```python
from build123d import *

# Parameters (mm, degrees)
SKETCH1_R            = 7.5
BOSS_EXTRUDE1_DEPTH  = 25
SKETCH4_R            = 7.5
BOSS_EXTRUDE4_DEPTH  = 40
BOSS_EXTRUDE4_TAPER  = 5
SKETCH5_R            = 2
BOSS_EXTRUDE5_DEPTH  = 1
SKETCH5_5_R          = 1.5
BOSS_EXTRUDE6_DEPTH  = 5
SKETCH6_R            = 2
BOSS_EXTRUDE7_DEPTH  = 1
SKETCH8_R            = 1.5
BOSS_EXTRUDE8_DEPTH  = 1
SKETCH9_R            = 2
BOSS_EXTRUDE9_DEPTH  = 1
SKETCH10_W           = 0.5
SKETCH10_H           = 3
BOSS_EXTRUDE10_DEPTH = 2
SKETCH11_W           = 0.5
SKETCH11_H           = 2
BOSS_EXTRUDE11_DEPTH = 15
SKETCH14_R           = 7.5
BOSS_EXTRUDE13_DEPTH = 10
BOSS_EXTRUDE13_TAPER = 10
SCALE1_SCALE         = 1.6


with BuildPart() as part:
    # Sketch1 → Boss-Extrude1 (new, symmetric)
    with BuildSketch(Plane.XY):
        Circle(SKETCH1_R)
    extrude(amount=BOSS_EXTRUDE1_DEPTH, both=True)

    # Sketch4 → Boss-Extrude4 (add)
    with BuildSketch(Plane.XY.offset(25)):
        Circle(SKETCH4_R)
    extrude(amount=BOSS_EXTRUDE4_DEPTH, taper=BOSS_EXTRUDE4_TAPER)

    # Sketch5 → Boss-Extrude5 (add)
    with BuildSketch(Plane.XY.offset(65)):
        Circle(SKETCH5_R)
    extrude(amount=BOSS_EXTRUDE5_DEPTH)

    # Sketch5<5> → Boss-Extrude6 (add)
    with BuildSketch(Plane.XY.offset(65)):
        Circle(SKETCH5_5_R)
    extrude(amount=BOSS_EXTRUDE6_DEPTH)

    # Sketch6 → Boss-Extrude7 (add)
    with BuildSketch(Plane.XY.offset(70)):
        Circle(SKETCH6_R)
    extrude(amount=BOSS_EXTRUDE7_DEPTH)

    # Sketch8 → Boss-Extrude8 (add)
    with BuildSketch(Plane.XY.offset(71)):
        Circle(SKETCH8_R)
    extrude(amount=BOSS_EXTRUDE8_DEPTH)

    # Sketch9 → Boss-Extrude9 (add)
    with BuildSketch(Plane.XY.offset(72)):
        Circle(SKETCH9_R)
    extrude(amount=BOSS_EXTRUDE9_DEPTH)

    # Sketch10 → Boss-Extrude10 (add)
    with BuildSketch(Plane.XY.offset(73)):
        Rectangle(SKETCH10_W, SKETCH10_H)
    extrude(amount=BOSS_EXTRUDE10_DEPTH)

    # Sketch11 → Boss-Extrude11 (add)
    with BuildSketch(Plane.XY.offset(75)):
        Rectangle(SKETCH11_W, SKETCH11_H)
    extrude(amount=BOSS_EXTRUDE11_DEPTH)

    # Sketch12 → Revolve1 (revolve)
    with BuildSketch(Plane(origin=(0, 0, 0), x_dir=(0, 0, -1), z_dir=(1, 0, 0))):
        with BuildLine():
            Line((-90, 0), (-93, 0))
            ThreePointArc((-93, 0), (-92.121320344, 2.121320344), (-90, 3))
            Line((-90, 3), (-90, 0))
        make_face()
    revolve(axis=Axis((0, 0, 90), (0, 0, 1)))

    # Sketch14 → Boss-Extrude13 (add)
    with BuildSketch(Plane(origin=(0, 0, -25), x_dir=(-1, 0, 0), z_dir=(0, 0, -1))):
        Circle(SKETCH14_R)
    extrude(amount=BOSS_EXTRUDE13_DEPTH, taper=BOSS_EXTRUDE13_TAPER)


with BuildPart() as part_1:
    # Scale1: scaled about (0, 0, 10.008668497)
    add(part.part.scale(SCALE1_SCALE).moved(Location((0, 0, -6.005201098))))


solid = part_1.part
```
For this review, take the finished solid that the model builds, in its own axes (mm). A direction names the side the tool comes from. Round coordinates to 2 decimals unless told otherwise and drop trailing zeros. Write each loop counter-clockwise with the first axis right and the second up, starting at its lowest first coordinate (ties: lowest second). Pieces come first, ordered by that corner, then holes. Notation, with made-up numbers: (64, 60.5) -> (87, 60.5) arc R36 ccw to (87, 99.5) -> close; hole circle Ø10 at (45.25, 50). An arc over 180 degrees is marked (long way). One line per question, with ' | ' between items. Start each with the question number.
1) Add section A-A (z = 116). Write out the cut boundary in (x, y), and give its area (3 significant figures).
2) Wall thickness on line 1 along Z through (x, y) = (-1.5, 2); line 2 along Z through (x, y) = (-1.25, 3.25); line 3 along Z through (x, y) = (5, -1): over which ranges is each line inside the solid? List them lowest first.
3) Machinability: for faces 1 (the cylindrical face through (-2.539, -1.947, 98.784)), 2 (the flat face through (0, 0, -62.005)), 3 (the flat face through (0.4, 0, 124)), which of the approach directions +Z, -Z, +X, -X, +Y, -Y give a long, thin tool a straight path to every point of the face, cutting with its end or side? Answer none if there is none.
4) For pin 1 Ø6 at (x, z) = (-8, 83.5) entering from +Y; pin 2 Ø3 at (x, y) = (2.5, -7) entering from +Z; pin 3 Ø0.6 at (x, z) = (0, 120) entering from -Y; pin 4 Ø8 at (y, z) = (-8, 107) entering from +X, all flat-tipped, find the tip position at first contact; note any pin that passes through.
5) Add section C-C (z = 36.5). Write out the cut boundary in (x, y), and give its area (3 significant figures).
6) Add section B-B (z = -25). Write out the cut boundary in (x, y).
7) Mouldability with a two-part tool opening along Z and no side actions: class faces 4 (the conical face through (8.14, -6.24, -55.89)), 5 (the cylindrical face through (-11.99, 0.53, -5.45)), 6 (the flat face through (-3, 2, 97.995)), 7 (the flat face through (-0.4, 0, 124)) as +Z half, -Z half, draft (parallel to the pull), parting line (faces both ways), or undercut.
Reported:
1) outline: (-0.4, -1.6) -> (0.4, -1.6) -> (0.4, 1.6) -> (-0.4, 1.6) -> close | area: 2.56 mm²
2) line 1: z = -62.01 to 99.59, 105.99 to 107.59, 109.19 to 110.79, 137.99 to 142.09 | line 2: z = -62.01 to 97.99, 137.99 to 141.3 | line 3: z = -62.01 to 97.99
3) face 1: none | face 2: -Z, +X, -X, +Y, -Y | face 3: +X, +Y, -Y
4) pin 1: stops at y = 5.84 | pin 2: stops at z = 97.99 | pin 3: stops at y = -1.6 | pin 4: passes through
5) outline: circle Ø23.56 at (0, 0) | area: 436 mm²
6) outline: circle Ø24 at (0, 0)
7) face 4: -Z half | face 5: draft | face 6: undercut | face 7: undercut
